Check sheet for the modelled part. Datum: model origin and axes. Units: mm. Face numbers are marked on the shaded views. A direction names the side the tool comes from. Round coordinates to 2 decimals unless told otherwise and drop trailing zeros. Write each loop counter-clockwise with the first axis right and the second up, starting at its lowest first coordinate (ties: lowest second). Pieces come first, ordered by that corner, then holes.
Item 1: Section check C-C, the plane z = 1.55. State how many separate pieces and enclosed holes the cut face has, plus the area to 3 significant figures.
Item 2: Set-up check for the marked faces 1, 2 and 3: record each of +Z, -Z, +X, -X, +Y, -Y from which the full face is reachable in a straight line by a thin tool's end or side.
Item 3: Section check D-D, the plane x = 225.25. Record the cut outline in (y, z).
Item 4: Material ranges on line 1 along Y through (x, z) = (227.5, 0.75); line 2 along X through (y, z) = (6.25, 1); line 3 along X through (y, z) = (-8.25, 1.25), recorded low to high.
Item 5: Section check A-A, the plane x = 223.75. Record the cut outline in (y, z).
Item 6: Section check B-B, the plane y = -6.25. Record the cut outline in (x, z).
Item 7: Release check for a two-part mould opening along Y. For the marked faces 4, 5 and 6 record: pulls with the +Y half, pulls with the -Y half, needs draft (parallel to the pull), parting line crosses it, or undercut.
Autodesk Fusion 360 part; units mm, degrees
sketch "Sketch1" plane through (0, 0, 0) normal (0, 0, 1) x (1, 0, 0)
  line L0 (230, 0) -> (230, -6)
  line L1 (230, -6) -> (234, -6)
  line L2 (234, -6) -> (234, -10)
  line L3 (234, -10) -> (222, -10)
  line L4 (222, -10) -> (222, -6)
  line L5 (222, -6) -> (226, -6)
  line L6 (226, -6) -> (226, 0)
  line L7 (226, 0) -> (230, 0)
  line L8 (230, 6) -> (234, 6)
  line L9 (234, 6) -> (234, 10)
  line L10 (234, 10) -> (222, 10)
  line L11 (222, 10) -> (222, 6)
  line L12 (222, 6) -> (226, 6)
  line L13 (226, 6) -> (226, 0)
  line L14 (230, 0) -> (230, 6)
  line L15 (229, 0) -> (229, 7)
  line L16 (229, 7) -> (233, 7)
  line L17 (233, 7) -> (233, 9)
  line L18 (233, 9) -> (223, 9)
  line L19 (223, 9) -> (223, 7)
  line L20 (223, 7) -> (227, 7)
  line L21 (227, 7) -> (227, 0)
  line L22 (229, 0) -> (229, -7)
  line L23 (229, -7) -> (233, -7)
  line L24 (233, -7) -> (233, -9)
  line L25 (233, -9) -> (223, -9)
  line L26 (223, -9) -> (223, -7)
  line L27 (223, -7) -> (227, -7)
  line L28 (227, -7) -> (227, 0)
  line L29 (235, -5) -> (235, -11)
  line L30 (235, -11) -> (221, -11)
  line L31 (221, -11) -> (221, -5)
  line L32 (221, -5) -> (225, -5)
  line L33 (225, -5) -> (225, 0)
  line L34 (225, 5) -> (225, 0)
  line L35 (221, 5) -> (225, 5)
  line L36 (221, 11) -> (221, 5)
  line L37 (235, 11) -> (221, 11)
  line L38 (235, 5) -> (235, 11)
  line L39 (231, 5) -> (235, 5)
  line L40 (231, 0) -> (231, 5)
  line L41 (231, 0) -> (231, -5)
  line L42 (231, -5) -> (235, -5)
  dimension "d775" = 6
  dimension "d776" = 4
  dimension "d777" = 12
  dimension "d778" = 4
  dimension "d779" = 4
  dimension "d780" = 4
  dimension "d781" = -1
  dimension "d782" = 1
  dimension "d783" = 1
extrude "Extrude1" add sketch "Sketch1" along normal blind 4 contours L7 L22 L23 L24 L25 L26 L27 L28 | L7 L15 L16 L17 L18 L19 L20 L21 | L29 L30 L31 L32 L33 L34 L35 L36 L37 L38 L39 L40 L41 L42 makes body 1 at (227.6667, -8.3333, 0) makes body 2 at (226, -10.6667, 0)
extrude "Extrude2" add sketch "Sketch1" along normal blind 2 from surface at 2 contours L0 L1 L2 L3 L4 L5 L6 L7 L22 L23 L24 L25 L26 L27 L28 | L7 L8 L9 L10 L11 L12 L13 L14 L15 L16 L17 L18 L19 L20 L21 bodies 1 2
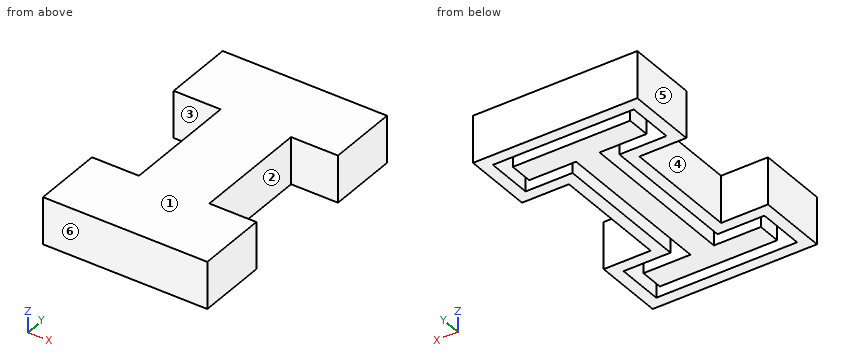
Values found:
1. separate pieces: 2
1. enclosed holes: 1
1. area: 152 mm2
2. face 1: +Z, +X, -X, +Y, -Y
2. face 2: +Z, -Z, +X
2. face 3: +Z, -Z, -X
3. outline: (-11, 0) - (-10, 0) - (-10, 2) - (-9, 2) - (-9, 0) - (-7, 0) - (-7, 2) - (-6, 2) - (-6, 0) - (6, 0) - (6, 2) - (7, 2) - (7, 0) - (9, 0) - (9, 2) - (10, 2) - (10, 0) - (11, 0) - (11, 4) - (-11, 4) - close
4. line 1: y = -11 to -10, -9 to 9, 10 to 11
4. line 2: x = 221 to 222, 227 to 229, 234 to 235
4. line 3: x = 221 to 222, 223 to 233, 234 to 235
5. outline: (-11, 0) - (-10, 0) - (-10, 2) - (-9, 2) - (-9, 0) - (-7, 0) - (-7, 2) - (-6, 2) - (-6, 0) - (-5, 0) - (-5, 4) - (-11, 4) - close; (5, 0) - (6, 0) - (6, 2) - (7, 2) - (7, 0) - (9, 0) - (9, 2) - (10, 2) - (10, 0) - (11, 0) - (11, 4) - (5, 4) - close
6. outline: (221, 0) - (222, 0) - (222, 2) - (227, 2) - (227, 0) - (229, 0) - (229, 2) - (234, 2) - (234, 0) - (235, 0) - (235, 4) - (221, 4) - close
7. face 4: undercut
7. face 5: needs draft
7. face 6: pulls with the -Y half
